Autodesk Inventor part; units mm, degrees
ref_plane "YZ Plane" through (0, 0, 0) normal (1, 0, 0) x (0, 1, 0)
ref_plane "XZ Plane" through (0, 0, 0) normal (0, 1, 0) x (-1, 0, 0)
ref_plane "XY Plane" through (0, 0, 0) normal (0, 0, 1) x (1, 0, 0)
sketch "Sketch1" plane through (0, 0, 0) normal (0, 1, 0) x (-1, 0, 0)
  line L0 (49.6769, 99.8505) -> (-26.5231, 99.8505)
  line L1 (-26.5231, 99.8505) -> (-26.5231, -46.1995)
  line L2 (-26.5231, -46.1995) -> (49.6769, -46.1995)
  line L3 (49.6769, -46.1995) -> (49.6769, 99.8505)
  point P0 (0, 0)
  dimension "d0" = 146.05
  dimension "d1" = 76.2
extrude "Extrusion1" add sketch "Sketch1" along normal blind 25.4
sketch "Sketch2" plane through (0, 25.4, 0) normal (0, 1, 0) x (1, 0, 0)
  circle A0 centre (-11.5769, -70.6659) radius 12.7
  line L0 (-49.6769, 46.1995) -> (-49.6769, -99.8505)
  line L1 (-49.6769, -99.8505) -> (26.5231, -99.8505)
  point P0 (0, 0)
  dimension "d4" = 25.4
  dimension "d5" = 38.1
  dimension "d6" = 29.1846
extrude "Extrusion2" cut sketch "Sketch2" against normal blind 25.4
sketch "Sketch3" plane through (0, 25.4, 0) normal (0, 1, 0) x (1, 0, 0)
  line L0 (-24.2769, 4.3149) -> (1.1231, 4.3149)
  line L1 (1.1231, 4.3149) -> (1.1231, 29.7149)
  line L2 (1.1231, 29.7149) -> (-24.2769, 29.7149)
  line L3 (-24.2769, 29.7149) -> (-24.2769, 4.3149)
  line L4 (26.5231, 46.1995) -> (-49.6769, 46.1995)
  line L5 (26.5231, -99.8505) -> (26.5231, 46.1995)
  point P0 (0, 0)
  dimension "d9" = 25.4
  dimension "d10" = 16.4846
  dimension "d11" = 25.4
extrude "Extrusion3" cut sketch "Sketch3" against normal blind 25.4
sketch "Sketch4" plane through (0, 25.4, 0) normal (0, 1, 0) x (1, 0, 0)
  line L0 (1.1231, -12.1697) -> (1.1231, -41.4813)
  line L1 (1.1231, -41.4813) -> (-24.2769, -26.7988)
  line L2 (-24.2769, -26.7988) -> (1.1231, -12.1697)
  line L3 (26.5231, 46.1995) -> (-49.6769, 46.1995)
  line L4 (26.5231, -99.8505) -> (26.5231, 46.1995)
  point P0 (0, 0)
  dimension "d14" = 25.4
  dimension "d15" = 29.3116
  dimension "d16" = 58.3692
  dimension "d17" = 25.4
extrude "Extrusion4" cut sketch "Sketch4" against normal blind 25.4
properties part number "Pegboard new"
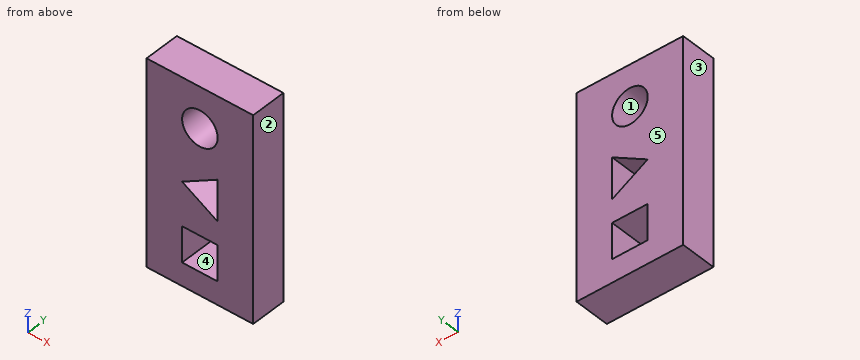
Model file for the job. Use its own axes, mm. Face numbers are marked on the shaded views. A direction names the side the tool comes from. Coordinates: 2 decimals unless noted, no trailing zeros. Loops run counter-clockwise (first coordinate to the right, second up) from the corner with the lowest first, then second, coordinate; pieces in that order, holes last. Notation, with made-up numbers: (22, 3) - (29, 3) arc R22 cw to (29, 19) - close; hole circle Ø10 at (-31.5, 0). An arc over 180 degrees is marked (long way). Write item = value, one per line. Start each with the question number.
Item 1: Saw through at A-A, the plane z = -28. List the corners of the cut face in (x, y), then the cut area to 3 significant figures.
Item 2: Saw through at D-D, the plane z = 18. List the corners of the cut face in (x, y), then the cut area to 3 significant figures.
Item 3: Pull direction X, two halves, no side cores. Call the marked faces 1, 2 and 3: +X half, -X half, draft (parallel to the pull), parting line (faces both ways), or undercut.
Item 4: Saw through at B-B, the plane x = -12. List the corners of the cut face in (y, z).
Item 5: Wall check: probe 1 along X at (y, z) = (10.5, -5); probe 2 along Z at (x, y) = (-7, 17.25); probe 3 along Z at (x, y) = (-23, 10.5). Give the ranges that are in metal, low to high. Write a range as [from, to].
Item 6: 3-axis set-ups, long thin cutter, end or side, ignore diameter. For the marked faces 4 and 5: which of +Z, -Z, +X, -X, +Y, -Y reach the whole face in a straight line?
Item 7: Saw through at C-C, the plane y = 6.25. List the corners of the cut face in (x, z).
Answers:
q1.outline = (-49.68, 0) - (-24.28, 0) - (-24.28, 25.4) - (-49.68, 25.4) - close; (1.12, 0) - (26.52, 0) - (26.52, 25.4) - (1.12, 25.4) - close
q1.area = 1,290 mm2
q2.outline = (-49.68, 0) - (-9, 0) - (-9, 25.4) - (-49.68, 25.4) - close; (1.12, 0) - (26.52, 0) - (26.52, 25.4) - (1.12, 25.4) - close
q2.area = 1,680 mm2
q3.face_1 = undercut
q3.face_2 = +X half
q3.face_3 = -X half
q4.outline = (0, -46.2) - (25.4, -46.2) - (25.4, -29.71) - (0, -29.71) - close; (0, -4.31) - (25.4, -4.31) - (25.4, 19.73) - (0, 19.73) - close; (0, 33.9) - (25.4, 33.9) - (25.4, 57.97) - (0, 57.97) - close; (0, 83.36) - (25.4, 83.36) - (25.4, 99.85) - (0, 99.85) - close
q5.probe_1 = [-49.68, -24.28], [1.12, 26.52]
q5.probe_2 = [-46.2, -29.71], [-4.31, 16.85], [36.79, 58.82], [82.51, 99.85]
q5.probe_3 = [-46.2, -29.71], [-4.31, 26.06], [27.54, 65.12], [76.22, 99.85]
q6.face_4 = +Y, -Y
q6.face_5 = +Z, -Z, +X, -X, +Y
q7.outline = (-49.68, -46.2) - (26.52, -46.2) - (26.52, 99.85) - (-49.68, 99.85) - close; hole (-24.28, -29.71) - (1.12, -29.71) - (1.12, -4.31) - (-24.28, -4.31) - close; hole (-24.28, 26.8) - (1.12, 12.17) - (1.12, 41.48) - close; hole circle Ø25.4 at (-11.58, 70.67)
